Here's how the part is built. I have some questions about the finished solid (model axes, mm). A direction names the side the tool comes from. Coordinates: 2 decimals unless noted, no trailing zeros. Order: outer loops, then holes, each group sorted by start corner. A loop starts at its lowest first (then second) coordinate and runs counter-clockwise, first axis right, second up. Notation, with made-up numbers: (-22.5, 76) - (6.5, 76) arc R13 ccw to (6.5, 93) - close; hole circle Ø9 at (11, -5). An arc over 180 degrees is marked (long way). Answer as CSV lines item,"result". Start each with the question number.
Item 1: On a 3-axis mill with a long thin cutter (end or side, diameter ignored), from which of +Z, -Z, +X, -X, +Y, -Y can I reach the whole of each face in a straight line? I mean faces 1 (the face through (22.225, 9, 4)), 2 (the face through (-33.43, -6.2, -1.38)), 3 (the face through (-23.812, -6, 0)). Say none if no direction works.
Item 2: I'm going to push flat-ended pins straight in: pin 1 (4 mm diameter, centred on x = 27.5, y = -5, fed in from +Z); pin 2 (3 mm diameter, centred on x = 11.5, z = 5, fed in from +Y); pin 3 (4 mm diameter, centred on y = 9.5, z = 9, fed in from -X). Where does each tip first touch, or does it pass through?
Item 3: Imagine slicing it at C-C on x = 33.5. List the corners of the cut face in (y, z) for me (1 decimal), and give its area (3 significant figures).
Item 4: Imagine slicing it at D-D on x = -34. List the corners of the cut face in (y, z) for me, and give its area (3 significant figures).
Item 5: I need wall thicknesses on line 1 (Y direction, x = 9.5, z = 5.5); line 2 (X direction, y = 10.25, z = 4.5) (3 decimals); line 3 (Z direction, x = 25, y = -5.5). Which ranges of each line are inside material? Lowest first, please.
from build123d import *

# Parameters (mm, degrees)
SKETCH2_R                = 12.7
BOSS_EXTRUDE1_DEPTH      = 39.6875
BOSS_EXTRUDE1_DEPTH_BACK = 39.6875
SKETCH3_OUTSIDE_W        = 44.824
SKETCH3_OUTSIDE_H        = 44.824
SKETCH3_OUTSIDE_R        = 7.9375
CUT_EXTRUDE1_DEPTH       = 17.4625
FILLET1_R                = 3.175
FILLET2_R                = 1.5875
CHAMFER1_SIZE            = 1.27
SKETCH4_OUTSIDE_W        = 44.824
SKETCH4_OUTSIDE_H        = 44.824
SKETCH4_OUTSIDE_R        = 6.35
CUT_EXTRUDE2_DEPTH       = 12.7
SKETCH6_OUTSIDE_W        = 44.824
SKETCH6_OUTSIDE_H        = 44.824
SKETCH6_OUTSIDE_R        = 5.588
CUT_EXTRUDE3_DEPTH       = 3.175
FILLET3_R                = 1.27
CHAMFER2_SIZE            = 0.762


with BuildPart() as part:
    # Sketch2 → Boss-Extrude1 (new body, two sides)
    with BuildSketch(Plane(origin=(0, 0, 0), x_dir=(0, 0, -1), z_dir=(1, 0, 0))) as boss_extrude1_sk:
        Circle(SKETCH2_R)
    extrude(amount=BOSS_EXTRUDE1_DEPTH)
    extrude(boss_extrude1_sk.sketch, amount=-BOSS_EXTRUDE1_DEPTH_BACK)

    # Sketch3 outside → Cut-Extrude1 (cut)
    with BuildSketch(Plane(origin=(39.6875, 0, 0), x_dir=(0, 0, -1), z_dir=(1, 0, 0))):
        Rectangle(SKETCH3_OUTSIDE_W, SKETCH3_OUTSIDE_H)
        Circle(SKETCH3_OUTSIDE_R, mode=Mode.SUBTRACT)
    extrude(amount=-CUT_EXTRUDE1_DEPTH, mode=Mode.SUBTRACT)

    # Fillet1
    fillet1_edges = [part.edges().sort_by_distance(p)[0] for p in [
        (39.6875, 0, 7.9375),
    ]]
    fillet(fillet1_edges, radius=FILLET1_R)

    # Fillet2
    fillet2_edges = [part.edges().sort_by_distance(p)[0] for p in [
        (22.225, 0, 7.9375),
    ]]
    fillet(fillet2_edges, radius=FILLET2_R)

    # Chamfer1
    chamfer1_edges = [part.edges().sort_by_distance(p)[0] for p in [
        (22.225, 0, 12.7),
    ]]
    chamfer(chamfer1_edges, length=CHAMFER1_SIZE)

    # Sketch4 outside → Cut-Extrude2 (cut)
    with BuildSketch(Plane.ZY.offset(39.6875)):
        Rectangle(SKETCH4_OUTSIDE_W, SKETCH4_OUTSIDE_H)
        Circle(SKETCH4_OUTSIDE_R, mode=Mode.SUBTRACT)
    extrude(amount=-CUT_EXTRUDE2_DEPTH, mode=Mode.SUBTRACT)

    # Sketch6 outside → Cut-Extrude3 (cut)
    with BuildSketch(Plane.ZY.offset(26.9875)):
        Rectangle(SKETCH6_OUTSIDE_W, SKETCH6_OUTSIDE_H)
        Circle(SKETCH6_OUTSIDE_R, mode=Mode.SUBTRACT)
    extrude(amount=-CUT_EXTRUDE3_DEPTH, mode=Mode.SUBTRACT)

    # Sketch13 → Cut-Revolve1 (revolve, cut)
    with BuildSketch(Plane.XY):
        Polygon((-23.8125, 6.35), (-12.7, 9.525), (-12.7, 12.7), (-23.8125, 12.7), align=None)
    revolve(axis=Axis((-43.65625, 0, 0), (1, 0, 0)), mode=Mode.SUBTRACT)

    # Fillet3
    fillet3_edges = [part.edges().sort_by_distance(p)[0] for p in [
        (-12.7, -9.525, 0),
    ]]
    fillet(fillet3_edges, radius=FILLET3_R)

    # Chamfer2
    chamfer2_edges = [part.edges().sort_by_distance(p)[0] for p in [
        (-12.7, 0, 12.7),
    ]]
    chamfer(chamfer2_edges, length=CHAMFER2_SIZE)


solid = part.part
Responses:
1,face 1,"+X"
1,face 2,"-X"
1,face 3,"none"
2,pin 1,"stops at z = 7.35"
2,pin 2,"stops at y = 12.21"
2,pin 3,"stops at x = -12.7"
3,outline,"circle Ø15.9 at (0, 0)"
3,area,"198 mm^2"
4,outline,"circle Ø12.7 at (0, 0)"
4,area,"127 mm^2"
5,line 1,"y = -11.45 to 11.45"
5,line 2,"x = -12.7 to 22.225"
5,line 3,"z = -5.72 to 5.72"
